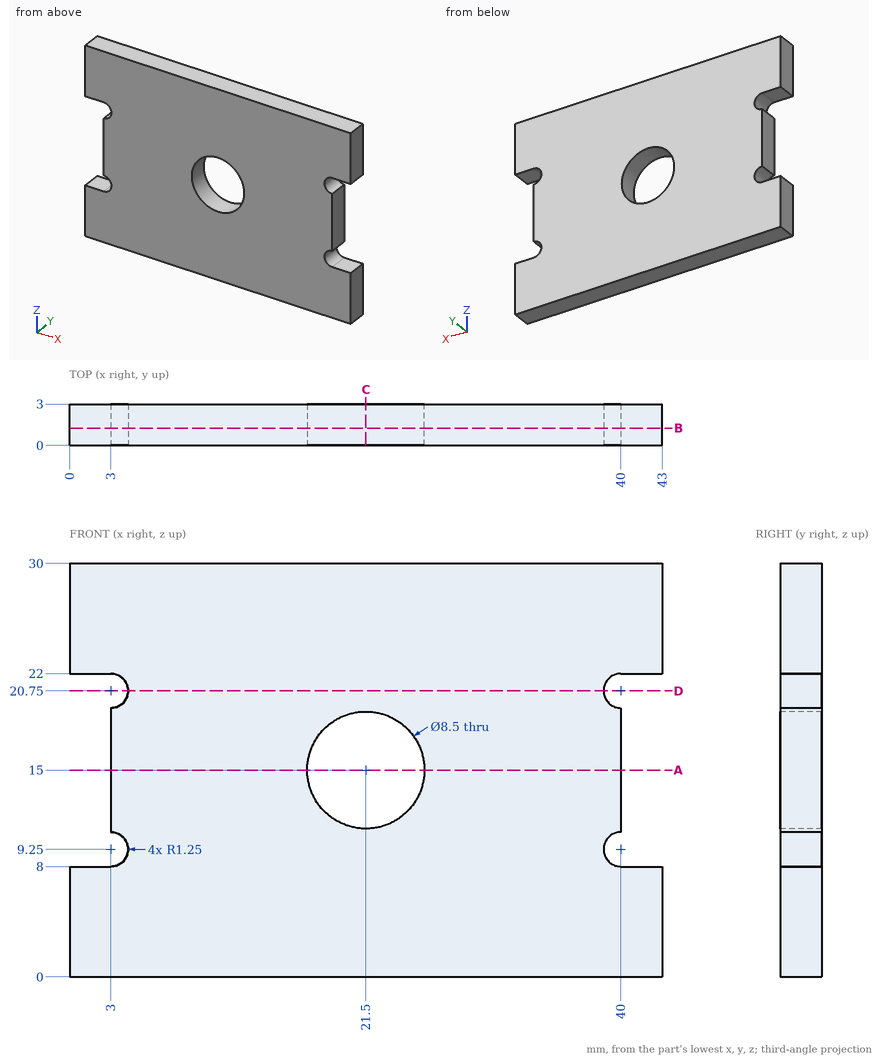
Geometry: see drawing. Coordinates: mm, zero at the bounding-box minimum. Round coordinates to 2 decimals unless told otherwise and drop trailing zeros. Order: outer loops, then holes, each group sorted by start corner. A loop starts at its lowest first (then second) coordinate and runs counter-clockwise, first axis right, second up. Notation, with made-up numbers: (49.25, 75.5) - (71.25, 75.5) arc R31 cw to (71.25, 113.5) - close; hole circle Ø6 at (-35, 23). An arc over 180 degrees is marked (long way). One line per question, with ' | ' between items. Start each with the question number.
1) Cut plane B-B, the plane y = 1.25. Return the cut outline in (x, z), then the cut area to 3 significant figures.
2) Cut plane C-C, the plane x = 21.5. Return the cut outline in (y, z).
3) Contact query for a flat-ended pin moving along its axis: P1, Ø1.5, axis at y = 1.5, z = 16, coming from the +X side. Output: stop coordinate, or through.
4) Ray query, probe 1 along Z at (x, y) = (21.5, 1.1); probe 2 along X at (y, z) = (1.7, 15); probe 3 along X at (y, z) = (1.8, 18). Return the intervals inside material, ascending.
5) Cut plane A-A, the plane z = 15. Return the cut outline in (x, y), then the cut area to 3 significant figures.
6) Cut plane D-D, the plane z = 20.75. Return the cut outline in (x, y).
Worked out:
1) outline: (0, 0) - (43, 0) - (43, 8) - (40, 8) arc R1.25 cw to (40, 10.5) - (40, 19.5) arc R1.25 cw to (40, 22) - (43, 22) - (43, 30) - (0, 30) - (0, 22) - (3, 22) arc R1.25 cw to (3, 19.5) - (3, 10.5) arc R1.25 cw to (3, 8) - (0, 8) - close; hole circle Ø8.5 at (21.5, 15) | area: 1,140 mm^2
2) outline: (0, 0) - (3, 0) - (3, 10.75) - (0, 10.75) - close; (0, 19.25) - (3, 19.25) - (3, 30) - (0, 30) - close
3) P1: stops at x = 40
4) probe 1: z = 0 to 10.75, 19.25 to 30 | probe 2: x = 3 to 17.25, 25.75 to 40 | probe 3: x = 3 to 18.49, 24.51 to 40
5) outline: (3, 0) - (17.25, 0) - (17.25, 3) - (3, 3) - close; (25.75, 0) - (40, 0) - (40, 3) - (25.75, 3) - close | area: 85.5 mm^2
6) outline: (4.25, 0) - (38.75, 0) - (38.75, 3) - (4.25, 3) - close
